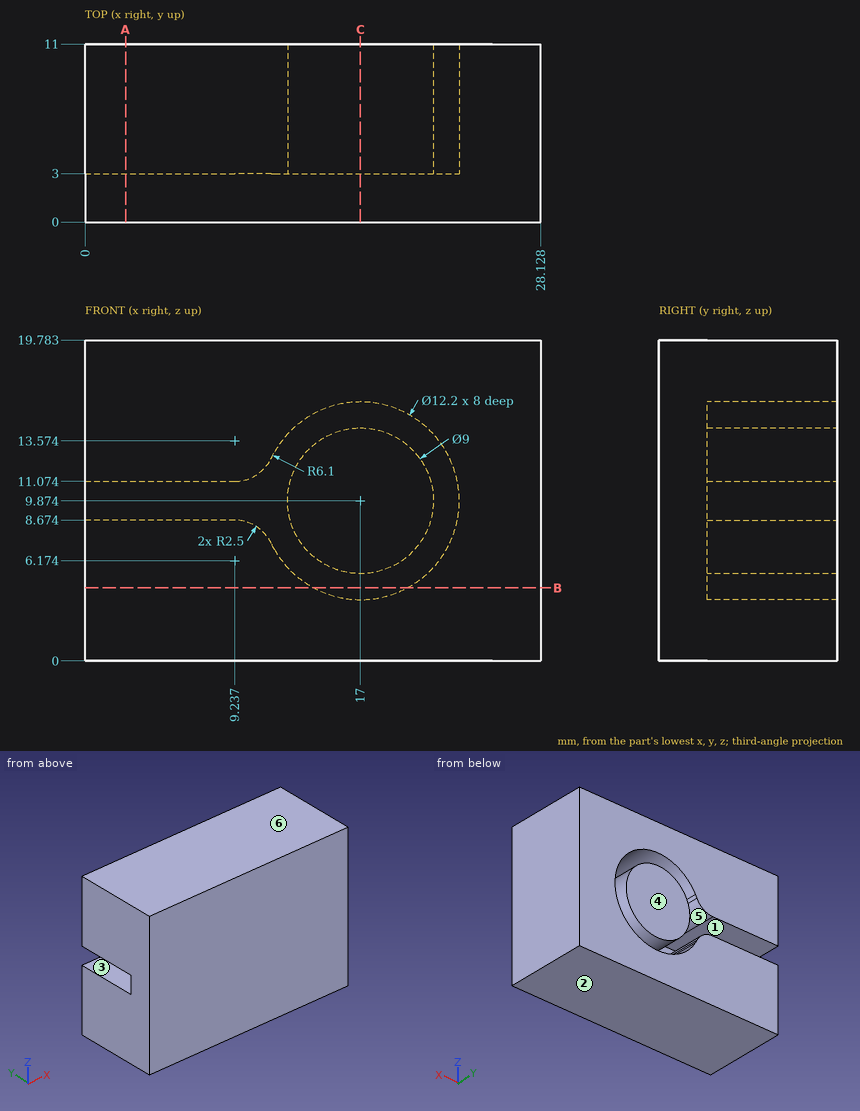
Geometry check sheet. Reference: drawing and pictorial views, mm from the part's lowest x, y, z. A direction names the side the tool comes from. Round coordinates to 2 decimals unless told otherwise and drop trailing zeros. Loops run counter-clockwise (first coordinate to the right, second up) from the corner with the lowest first, then second, coordinate; pieces in that order, holes last. Notation, with made-up numbers: (37, 76) - (44, 76) arc R26 ccw to (44, 98) - close; hole circle Ø7 at (63, 10.25). An arc over 180 degrees is marked (long way). Answer in a Markdown table with one row per item. Add a question column.
Q1. Tool access check on the marked faces 5 and 6. Record the directions out of +Z, -Z, +X, -X, +Y, -Y that give a thin tool (end or side, any length) a straight path to the whole face; none if there is none.
Q2. Gauge pin test, flat end, axial feed: pin 1 (7.5 mm diameter, centred on x = 17, z = 9.87, fed in from -Y). Record the tip position at first contact, or that the pin passes through.
Q3. Release check for a two-part mould opening along Z. For the marked faces 1, 2, 3 and 4 record: pulls with the +Z half, pulls with the -Z half, needs draft (parallel to the pull), parting line crosses it, or undercut.
Q4. Section check C-C on x = 17. Enter the section's corners in (y, z) (1 decimal), plus the area to 3 significant figures.
Q5. Section check A-A on x = 2.5. Enter the section's corners in (y, z) (1 decimal), plus the area to 3 significant figures.
Q6. Material ranges on line 1 (X direction, y = 8, z = 6.5) (1 decimal); line 2 (X direction, y = 5, z = 7.5) (1 decimal); line 3 (Z direction, x = 1.75, y = 3.25) (1 decimal), recorded low to high.
Q7. Section check B-B on z = 4.5. Enter the section's corners in (x, y) (1 decimal).
Found:
| question | item | result |
|---|---|---|
| 1 | face 5 | +Y |
| 1 | face 6 | +Z, +X, -X, +Y, -Y |
| 2 | pin 1 | stops at y = 0 |
| 3 | face 1 | undercut |
| 3 | face 2 | pulls with the -Z half |
| 3 | face 3 | undercut |
| 3 | face 4 | needs draft |
| 4 | outline | (0, 0) - (11, 0) - (11, 3.8) - (3, 3.8) - (3, 5.4) - (11, 5.4) - (11, 14.4) - (3, 14.4) - (3, 16) - (11, 16) - (11, 19.8) - (0, 19.8) - close |
| 4 | area | 192 mm² |
| 5 | outline | (0, 0) - (11, 0) - (11, 8.7) - (3, 8.7) - (3, 11.1) - (11, 11.1) - (11, 19.8) - (0, 19.8) - close |
| 5 | area | 198 mm² |
| 6 | line 1 | x = 0 to 11.9, 14 to 20, 22.1 to 28.1 |
| 6 | line 2 | x = 0 to 11.4, 13.2 to 20.8, 22.6 to 28.1 |
| 6 | line 3 | z = 0 to 8.7, 11.1 to 19.8 |
| 7 | outline | (0, 0) - (28.1, 0) - (28.1, 11) - (19.9, 11) - (19.9, 3) - (14.1, 3) - (14.1, 11) - (0, 11) - close |
